The figure shows three views and two pictorial views of one solid part (mm, origin at its lowest corner). Answer the questions. A direction names the side the tool comes from. Round coordinates to 2 decimals unless told otherwise and drop trailing zeros. Order: outer loops, then holes, each group sorted by start corner. A loop starts at its lowest first (then second) coordinate and runs counter-clockwise, first axis right, second up. Notation, with made-up numbers: (26, 74.5) - (46, 74.5) arc R17 ccw to (46, 93.5) - close; hole circle Ø4 at (-14.5, 88). An arc over 180 degrees is marked (long way). Use CSV: the item, a comma, the result in double quotes. Start each with the question number.
Item 1: For the marked faces 1 and 2, determine the directions among +Z, -Z, +X, -X, +Y, -Y from which every point of the face is accessible in a straight line to the end or side of a thin tool.
Item 2: Flat-ended cylindrical pins translate along their axes: P1, Ø1.8, axis at x = 36.5, y = 5.5, coming from the +Z side; P2, Ø12, axis at x = 20, y = 8.5, coming from the +Z side; P3, Ø2.5, axis at x = 5.5, y = 5.5, coming from the +Z side. Find the tip coordinate at first contact, or state that the pin passes through.
Item 3: Find section A-A, the plane x = 21. Give the vertices of the cut face in (y, z), plus the area to 4 significant figures.
Item 4: Find section D-D, the plane y = 30.5. Give the vertices of the cut face in (x, z) (1 decimal).
Item 5: Straight lines are drawn through the part: line 1 along Y through (x, z) = (36.5, 43); line 2 along X through (y, z) = (5, 46) (1 decimal). For each, find the intervals that lie inside material, in ascending order. Write a range as [from, to].
Item 6: Find section C-C, the plane z = 68. Give the vertices of the cut face in (x, y), plus the area to 3 significant figures.
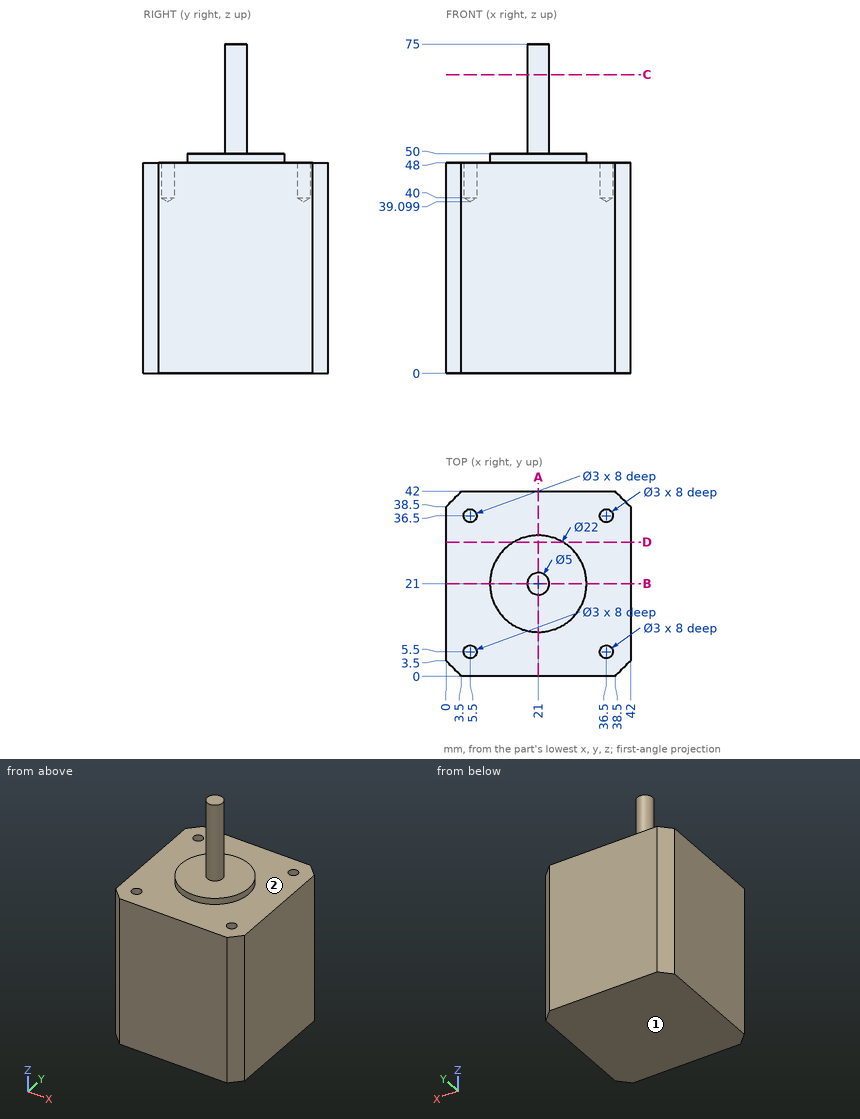
Worked out:
1,face 1,"-Z, +X, -X, +Y, -Y"
1,face 2,"+Z"
2,P1,"stops at z = 39.64"
2,P2,"stops at z = 50"
2,P3,"stops at z = 39.85"
3,outline,"(0, 0) - (42, 0) - (42, 48) - (32, 48) - (32, 50) - (23.5, 50) - (23.5, 75) - (18.5, 75) - (18.5, 50) - (10, 50) - (10, 48) - (0, 48) - close"
3,area,"2,185 mm²"
4,outline,"(0, 0) - (42, 0) - (42, 48) - (26.5, 48) - (26.5, 50) - (15.5, 50) - (15.5, 48) - (0, 48) - close"
5,line 1,"y = [0, 4], [7, 35], [38, 42]"
5,line 2,"x = [0, 4.1], [6.9, 35.1], [37.9, 42]"
6,outline,"circle Ø5 at (21, 21)"
6,area,"19.6 mm²"
